from build123d import *

# Parameters (mm, degrees)
BOSS_EXTRUDE1_DEPTH = 5
SKETCH2_R           = 2.1
CUT_EXTRUDE1_DEPTH  = 6


with BuildPart() as part:
    # Sketch1 → Boss-Extrude1 (new body, symmetric)
    with BuildSketch(Plane.XY):
        Polygon((-5, 1.5), (-5, -0.5), (-3, -2.5), (3, -2.5), (5, -0.5), (5, 1.5), (3, 1.5), (3, 2.5), (-3, 2.5), (-3, 1.5), align=None)
    extrude(amount=BOSS_EXTRUDE1_DEPTH, both=True)

    # Sketch2 → Cut-Extrude1 (cut, through all)
    with BuildSketch(Plane(origin=(0, 2.5, 0), x_dir=(1, 0, 0), z_dir=(0, 1, 0))):
        Circle(SKETCH2_R)
    extrude(amount=-CUT_EXTRUDE1_DEPTH, mode=Mode.SUBTRACT)


solid = part.part
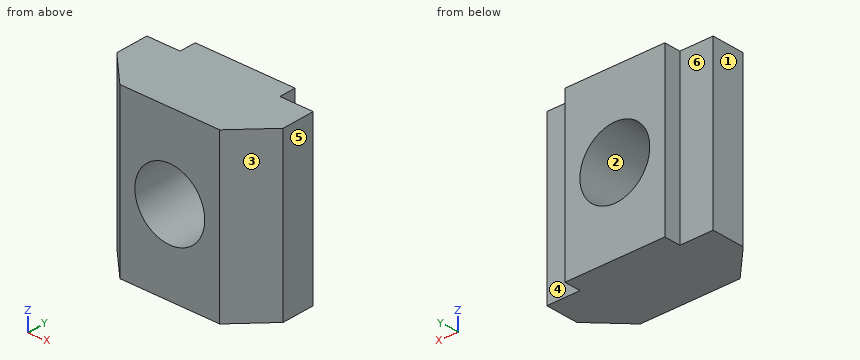
Model file for the job. Use its own axes, mm. Face numbers are marked on the shaded views. A direction names the side the tool comes from. Give positions to 0.01 mm unless a question says otherwise; leave off trailing zeros. Order: outer loops, then holes, each group sorted by start corner. A loop starts at its lowest first (then second) coordinate and runs counter-clockwise, first axis right, second up. Notation, with made-up numbers: (-38.5, 62) -> (-19.5, 62) arc R22 cw to (-19.5, 72) -> close; hole circle Ø3 at (54.5, -11). An arc over 180 degrees is marked (long way). Use CSV: the item, a comma, the result in double quotes.
1. Band-saw the part on C-C, the plane y = -1.3. Give the cut face in (x, z), then the cut area to 3 significant figures.
Outcome:
outline,"(-4.2, -5) -> (4.2, -5) -> (4.2, 5) -> (-4.2, 5) -> close; hole circle Ø4.2 at (0, 0)"
area,"70.1 mm²"
2. Band-saw the part on B-B, the plane x = 0. Give the cut face in (y, z), then the cut area to 3 significant figures.
Outcome:
outline,"(-2.5, -5) -> (2.5, -5) -> (2.5, -2.1) -> (-2.5, -2.1) -> close; (-2.5, 2.1) -> (2.5, 2.1) -> (2.5, 5) -> (-2.5, 5) -> close"
area,"29.0 mm²"
3. Drop flat-ended pins along their axis: pin 1 (1 mm diameter, centred on x = -4, z = -0.5, fed in from +Y); pin 2 (0.5 mm diameter, centred on y = 2, z = -0.5, fed in from -X); pin 3 (2.5 mm diameter, centred on x = 0, z = 0, fed in from +Y). Give the stop position or say it passes through.
Outcome:
pin 1,"y = 1.5"
pin 2,"x = -3"
pin 3,"through"
4. Drill centre lines: line 1 along X through (y, z) = (0.5, 0); line 2 along Z through (x, y) = (-1, 1.6). Where is each one in solid material? Low to high. Write a range as from..to.
Outcome:
line 1,"-5..-2.1, 2.1..5"
line 2,"-5..-1.85, 1.85..5"
5. Mould opens along X. For the marked faces 1, 2, 3 and 4 say: +X half, -X half, draft (parallel to the pull), parting line (faces both ways), or undercut.
Outcome:
face 1,"-X half"
face 2,"undercut"
face 3,"+X half"
face 4,"draft"
6. Band-saw the part on D-D, the plane z = 4.25. Give the cut face in (x, y).
Outcome:
outline,"(-5, -0.5) -> (-3, -2.5) -> (3, -2.5) -> (5, -0.5) -> (5, 1.5) -> (3, 1.5) -> (3, 2.5) -> (-3, 2.5) -> (-3, 1.5) -> (-5, 1.5) -> close"
7. Band-saw the part on A-A, the plane z = 0. Give the cut face in (x, y).
Outcome:
outline,"(-5, -0.5) -> (-3, -2.5) -> (-2.1, -2.5) -> (-2.1, 2.5) -> (-3, 2.5) -> (-3, 1.5) -> (-5, 1.5) -> close; (2.1, -2.5) -> (3, -2.5) -> (5, -0.5) -> (5, 1.5) -> (3, 1.5) -> (3, 2.5) -> (2.1, 2.5) -> close"
8. 3-axis set-ups, long thin cutter, end or side, ignore diameter. For the marked faces 5 and 6: which of +Z, -Z, +X, -X, +Y, -Y reach the whole face in a straight line?
Outcome:
face 5,"+Z, -Z, +X, +Y, -Y"
face 6,"+Z, -Z, -X, +Y"
